Could you check a few things on this model? Use its own coordinates, in mm. Coordinates: 2 decimals unless noted, no trailing zeros. Loops run counter-clockwise (first coordinate to the right, second up) from the corner with the lowest first, then second, coordinate; pieces in that order, holes last. Notation, with made-up numbers: (-24, 74) -> (-15, 74) arc R29 cw to (-15, 96) -> close; hole circle Ø6 at (-14.5, 44.25). An arc over 180 degrees is marked (long way). One line per question, with ' | ' between items. Start each with the question number.
(1) I'm going to push flat-ended pins straight in: pin 1 Ø2 at (x, y) = (15, -3) entering from -Z; pin 2 Ø3 at (x, y) = (-17.5, -3) entering from -Z. Where does each tip first touch, or does it pass through?
(2) If I drill on line 1 along Z through (x, y) = (-30.5, -4.6); line 2 along Y through (x, z) = (24.5, 31); line 3 along X through (y, z) = (-2.95, -29), over which ranges is the centre line in solid material (lowest first)?
(3) Suppose I cut it at A-A (y = -2.2). Please give me the cut outline in (x, z).
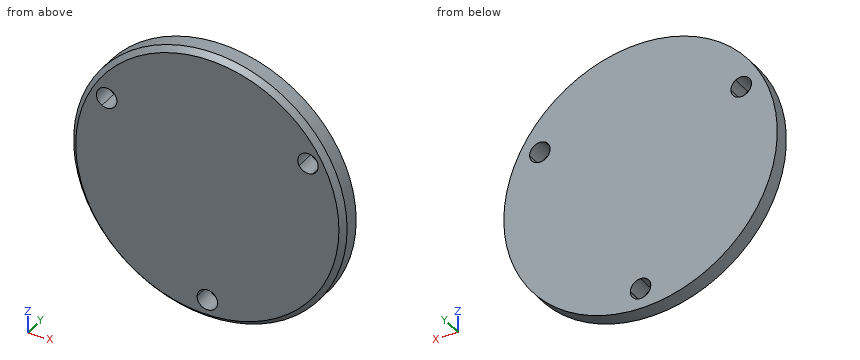
```python
from build123d import *

# Parameters (mm, degrees)
F0_R     = 40
F1_DEPTH = 6
F2_SIZE  = 1.5
F4_DEPTH = 25


with BuildPart() as f1:
    # F0 (on Front) → F1 (new body)
    with BuildSketch(Plane.XZ):
        Circle(F0_R)
    extrude(amount=F1_DEPTH)

    # F2
    f2_edges = [f1.edges().sort_by_distance(p)[0] for p in [
        (-40, -6, 0),
    ]]
    chamfer(f2_edges, length=F2_SIZE)

    # F3 (on face) → F4 (cut)
    with BuildSketch(Plane.XZ.offset(6)):
        with BuildLine():
            ThreePointArc((-29.444864, 17), (-28.666195, 18.282486), (-27.831703, 19.52937))
            ThreePointArc((-27.831703, 19.52937), (-32.04294, 18.5), (-30.828782, 14.338277))
            ThreePointArc((-30.828782, 14.338277), (-30.166195, 15.68441), (-29.444864, 17))
        make_face()
        with BuildLine():
            ThreePointArc((-30.828782, 14.338277), (-28.604658, 14.12006), (-26.846788, 15.5))
            Line((-26.846788, 15.5), (-29.444864, 17))
            ThreePointArc((-29.444864, 17), (-30.166195, 15.68441), (-30.828782, 14.338277))
        make_face()
        with BuildLine():
            ThreePointArc((-26.444864, 17), (-26.814324, 18.44231), (-27.831703, 19.52937))
            ThreePointArc((-27.831703, 19.52937), (-28.666195, 18.282486), (-29.444864, 17))
            Line((-29.444864, 17), (-26.846788, 15.5))
            ThreePointArc((-26.846788, 15.5), (-26.547086, 16.223543), (-26.444864, 17))
        make_face()
        with BuildLine():
            ThreePointArc((29.444864, 17), (30.166195, 15.68441), (30.828782, 14.338277))
            ThreePointArc((30.828782, 14.338277), (32.009211, 15.443041), (32.444864, 17))
            ThreePointArc((32.444864, 17), (30.887174, 19.63054), (27.831703, 19.52937))
            ThreePointArc((27.831703, 19.52937), (28.666195, 18.282486), (29.444864, 17))
        make_face()
        with BuildLine():
            ThreePointArc((26.846788, 15.5), (28.604658, 14.12006), (30.828782, 14.338277))
            ThreePointArc((30.828782, 14.338277), (30.166195, 15.68441), (29.444864, 17))
            Line((29.444864, 17), (26.846788, 15.5))
        make_face()
        with BuildLine():
            Line((26.846788, 15.5), (29.444864, 17))
            ThreePointArc((29.444864, 17), (28.666195, 18.282486), (27.831703, 19.52937))
            ThreePointArc((27.831703, 19.52937), (26.53066, 17.712331), (26.846788, 15.5))
        make_face()
        with BuildLine():
            ThreePointArc((-2.997079, -33.867647), (-1.5, -33.966896), (0, -34))
            Line((0, -34), (0, -31))
            ThreePointArc((0, -31), (-2.073999, -31.832391), (-2.997079, -33.867647))
        make_face()
        with BuildLine():
            ThreePointArc((0, -34), (1.5, -33.966896), (2.997079, -33.867647))
            ThreePointArc((2.997079, -33.867647), (2.073999, -31.832391), (0, -31))
            Line((0, -31), (0, -34))
        make_face()
        with BuildLine():
            ThreePointArc((3, -34), (2.99927, -33.933807), (2.997079, -33.867647))
            ThreePointArc((2.997079, -33.867647), (1.5, -33.966896), (0, -34))
            ThreePointArc((0, -34), (-1.5, -33.966896), (-2.997079, -33.867647))
            ThreePointArc((-2.997079, -33.867647), (-0.066193, -36.99927), (3, -34))
        make_face()
    extrude(amount=-F4_DEPTH, mode=Mode.SUBTRACT)


solid = f1.part
```
Checks:
1) pin 1: stops at z = -37.47 | pin 2: stops at z = -36.66
2) line 1: z = -25.72 to 14.19, 19.81 to 25.72 | line 2: y = -4.99 to 0 | line 3: x = -27.55 to 27.55
3) outline: circle Ø80 at (0, 0); hole (-30.83, 14.34) arc R3 ccw to (-26.85, 15.5) arc R3 ccw to (-26.44, 17) arc R3 ccw to (-27.83, 19.53) arc R3 ccw (long way) to start; hole (3, -34) arc R3 ccw to (3, -33.87) arc R3 ccw (long way) to start; hole (26.85, 15.5) arc R3 ccw to (30.83, 14.34) arc R3 ccw to (32.44, 17) arc R3 ccw (long way) to start
